CAD build for the part. Positions are in the model's coordinates, mm. A direction names the side the tool comes from. Round coordinates to 2 decimals unless told otherwise and drop trailing zeros. Loops run counter-clockwise (first coordinate to the right, second up) from the corner with the lowest first, then second, coordinate; pieces in that order, holes last. Notation, with made-up numbers: (83.5, 45.25) - (106.5, 45.25) arc R19 cw to (106.5, 61.25) - close; hole circle Ø6 at (50.25, 38). An arc over 180 degrees is marked (long way). Use one line per item in the form item = value.
from build123d import *

# Parameters (mm, degrees)
F0_W      = 720
F0_H      = 300
F1_DEPTH  = 25
F2_W      = 50
F2_H      = 50
F3_DEPTH  = 100
F4_W      = 50
F4_H      = 50
F5_DEPTH  = 100
F6_W      = 50
F6_H      = 50
F7_DEPTH  = 25
F8_R      = 25
F9_DEPTH  = 150
F10_W     = 45
F10_H     = 106.8337794484
F11_DEPTH = 150
F13_DEPTH = 50
F14_W     = 70
F14_H     = 70
F15_DEPTH = 150
F16_DEPTH = 130
F17_R     = 25
F18_W     = 150
F18_H     = 120
F19_DEPTH = 25
F20_W     = 60
F20_H     = 35
F21_DEPTH = 50
F23_DEPTH = 300
F24_W     = 104
F24_H     = 100
F25_DEPTH = 150
F26_W     = 104
F26_H     = 170
F27_DEPTH = 25
F28_W     = 29
F28_H     = 40
F29_DEPTH = 30
F30_W     = 150
F30_H     = 10
F31_DEPTH = 10


with BuildPart() as f1:
    # F0 (on Top) → F1 (new body)
    with BuildSketch(Plane.XY):
        Rectangle(F0_W, F0_H)
    extrude(amount=F1_DEPTH)

    # F2 (on face) → F3 (join)
    with BuildSketch(Plane.XY.offset(25)):
        with Locations((-335, -125)):
            Rectangle(F2_W, F2_H)
    extrude(amount=F3_DEPTH)

    # F4 (on face) → F5 (join)
    with BuildSketch(Plane.XY.offset(25)):
        with Locations((335, -125)):
            Rectangle(F4_W, F4_H)
        with Locations((-335, 125)):
            Rectangle(F4_W, F4_H)
        with Locations((335, 125)):
            Rectangle(F4_W, F4_H)
    extrude(amount=F5_DEPTH)

    # F6 (on face) → F7 (join)
    with BuildSketch(Plane.XY.offset(125)):
        with Locations((-335, 125)):
            Rectangle(F6_W, F6_H)
        Polygon((360, 150), (-310, 150), (-310, 100), (-360, 100), (-360, -150), (360, -150), align=None)
    extrude(amount=F7_DEPTH)

    # F8 (on face) → F9 (join)
    with BuildSketch(Plane.XY.offset(150)):
        with Locations((-310, 0)):
            Circle(F8_R)
    extrude(amount=F9_DEPTH)

    # F10 (on face) → F11 (join)
    with BuildSketch(Plane.XY.offset(150)):
        with Locations((106.5, -53.4168897242)):
            Rectangle(F10_W, F10_H)
        with Locations((106.5, 53.4168897242)):
            Rectangle(F10_W, F10_H)
    extrude(amount=F11_DEPTH)

    # F12 (on face) → F13 (cut)
    with BuildSketch(Plane.YZ.offset(129)):
        Polygon((81.8337794484, 300), (-81.8337794484, 300), (-81.8337794484, 221.9447493553), (-21.8337794484, 234.4899773598), (0, 209.3995064497), (21.8337794484, 234.4899773598), (81.8337794484, 221.9447493553), align=None)
    extrude(amount=-F13_DEPTH, mode=Mode.SUBTRACT)

    # F14 (on face) → F15 (join)
    with BuildSketch(Plane.XY.offset(150)):
        with Locations((221, 185)):
            Rectangle(F14_W, F14_H)
    extrude(amount=-F15_DEPTH)

    # F14 (on face) → F16 (join)
    with BuildSketch(Plane.XY.offset(150)):
        with Locations((221, 185)):
            Rectangle(F14_W, F14_H)
    extrude(amount=F16_DEPTH)

    # F17
    f17_edges = [f1.edges().sort_by_distance(p)[0] for p in [
        (-335, 0, 300),
    ]]
    fillet(f17_edges, radius=F17_R)

    # F18 (on face) → F19 (cut)
    with BuildSketch(Plane.XY.offset(150)):
        with Locations((285, -10)):
            Rectangle(F18_W, F18_H)
    extrude(amount=-F19_DEPTH, mode=Mode.SUBTRACT)

    # F20 (on face) → F21 (join)
    with BuildSketch(Plane.XY.offset(150)):
        with Locations((176.6629952192, -132.5)):
            Rectangle(F20_W, F20_H)
        with Locations((176.6629952192, 132.5)):
            Rectangle(F20_W, F20_H)
    extrude(amount=F21_DEPTH)

    # F22 (on face) → F23 (cut)
    with BuildSketch(Plane.XZ.offset(150)):
        with BuildLine():
            Line((191.6629952192, 200), (161.6629952192, 200))
            ThreePointArc((161.6629952192, 200), (176.6629952192, 185), (191.6629952192, 200))
        make_face()
    extrude(amount=-F23_DEPTH, mode=Mode.SUBTRACT)

    # F24 (on face) → F25 (cut)
    with BuildSketch(Plane.XY.offset(150)):
        with Locations((308, 100)):
            Rectangle(F24_W, F24_H)
    extrude(amount=-F25_DEPTH, mode=Mode.SUBTRACT)

    # F26 (on face) → F27 (join)
    with BuildSketch(Plane.XY.offset(25)):
        with Locations((308, 135)):
            Rectangle(F26_W, F26_H)
    extrude(amount=-F27_DEPTH)

    # F28 (on face) → F29 (join)
    with BuildSketch(Plane.YZ.offset(256)):
        with Locations((205.5, 260)):
            Rectangle(F28_W, F28_H)
        with Locations((205.5, 45)):
            Rectangle(F28_W, F28_H)
    extrude(amount=F29_DEPTH)

    # F30 (on face) → F31 (join)
    with BuildSketch(Plane.XY.offset(25)):
        with Locations((285, -75)):
            Rectangle(F30_W, F30_H)
    extrude(amount=F31_DEPTH)


solid = f1.part
1) Slice it at B-B (x = -164). Write the cut outline in (y, z).
Report:
outline = (-150, 0) - (150, 0) - (150, 25) - (-150, 25) - close; (-150, 125) - (150, 125) - (150, 150) - (-150, 150) - close
2) Drill centre lines: probe 1 along Z at (x, y) = (21, -96); probe 2 along X at (y, z) = (-106, 93); probe 3 along X at (y, z) = (203.5, 163). Where is each one in solid material? Low to high.
Report:
probe_1 = 0 to 25, 125 to 150
probe_2 = -360 to -310, 310 to 360
probe_3 = 186 to 256
3) Slice it at C-C (y = 128.5). Write the cut outline in (x, z).
Report:
outline = (-360, 0) - (360, 0) - (360, 25) - (-310, 25) - (-310, 125) - (256, 125) - (256, 150) - (206.66, 150) - (206.66, 200) - (191.66, 200) arc R15 cw to (161.66, 200) - (146.66, 200) - (146.66, 150) - (-360, 150) - close
4) Flat gauge pins, fed straight in: pin 1 (17.5 mm diameter, centred on y = 131.5, z = 169.5, fed in from -X); pin 2 (16.5 mm diameter, centred on x = 157, y = 126.5, fed in from +Z); pin 3 (10.5 mm diameter, centred on y = 133, z = 164.5, fed in from +X). Where does each tip first touch, or does it go through?
Report:
pin_1 = 146.66
pin_2 = 200
pin_3 = 206.66
5) Two-plate mould, pull along X, no slides. Class faces 1 (the flat face through (-5, -150, 143)), 2 (the flat face through (310, -125, 74)), 3 (the flat face through (186, 185, 138)): +X half, -X half, draft (parallel to the pull), parting line (faces both ways), or undercut.
Report:
face_1 = draft
face_2 = undercut
face_3 = -X half
6) Slice it at D-D (z = 173). Write the cut outline in (x, y), plus the area to 3 significant figures.
Report:
outline = circle Ø50 at (-310, 0); (84, -106.83) - (129, -106.83) - (129, 106.83) - (84, 106.83) - close; (146.66, -150) - (206.66, -150) - (206.66, -115) - (146.66, -115) - close; (146.66, 115) - (206.66, 115) - (206.66, 150) - (256, 150) - (256, 220) - (186, 220) - (186, 150) - (146.66, 150) - close
area = 20,700 mm^2
7) Slice it at A-A (z = 257). Write the cut outline in (x, y).
Report:
outline = circle Ø50 at (-310, 0); (84, -106.83) - (129, -106.83) - (129, -81.83) - (84, -81.83) - close; (84, 81.83) - (129, 81.83) - (129, 106.83) - (84, 106.83) - close; (186, 150) - (256, 150) - (256, 191) - (286, 191) - (286, 220) - (186, 220) - close
8) Tool access for faces 4 (the flat face through (199, 133, 200)), 5 (the flat face through (271, 205, 65)), 6 (the flat face through (-129, 150, 18)), 7 (the flat face through (206.663, -133, 175)): list every direction of +Z, -Z, +X, -X, +Y, -Y with a clear straight run to the whole face (end or side of a thin tool).
Report:
face_4 = +Z, +X, -X, -Y
face_5 = +X, +Y, -Y
face_6 = +Z, -Z, -X, +Y
face_7 = +Z, +X, -Y
